from build123d import *

# Parameters (mm, degrees)
SKETCH1_R           = 2
SKETCH1_R_2         = 1.95
SKETCH1_R_3         = 1.5
BOSS_EXTRUDE1_DEPTH = 5
SKETCH2_R           = 1.5
SKETCH2_R_2         = 1.95
SKETCH2_R_3         = 2
SKETCH2_W           = 36
SKETCH2_H           = 70
CUT_EXTRUDE1_DEPTH  = 142.509716981
FILLET1_R           = 2


with BuildPart() as part:
    # Sketch1 → Boss-Extrude1 (new body)
    with BuildSketch(Plane.XY):
        with BuildLine():
            Line((-90, 100), (-70, 100))
            Line((-70, 100), (-14.884168151, 68.505238943))
            ThreePointArc((-14.884168151, 68.505238943), (0, 64.552533207), (14.884168151, 68.505238943))
            Line((14.884168151, 68.505238943), (70, 100))
            Line((70, 100), (90, 100))
            ThreePointArc((90, 100), (97.071067812, 97.071067812), (100, 90))
            Line((100, 90), (100, 29))
            Line((100, 29), (93.372317414, 9.7797205))
            ThreePointArc((93.372317414, 9.7797205), (91.733506862, 0), (93.372317414, -9.7797205))
            Line((93.372317414, -9.7797205), (100, -29))
            Line((100, -29), (100, -90))
            ThreePointArc((100, -90), (97.071067812, -97.071067812), (90, -100))
            Line((90, -100), (70, -100))
            Line((70, -100), (14.884168151, -68.505238943))
            ThreePointArc((14.884168151, -68.505238943), (0, -64.552533207), (-14.884168151, -68.505238943))
            Line((-14.884168151, -68.505238943), (-70, -100))
            Line((-70, -100), (-90, -100))
            ThreePointArc((-90, -100), (-97.071067812, -97.071067812), (-100, -90))
            Line((-100, -90), (-100, -29))
            Line((-100, -29), (-93.372317414, -9.7797205))
            ThreePointArc((-93.372317414, -9.7797205), (-91.733506862, 0), (-93.372317414, 9.7797205))
            Line((-93.372317414, 9.7797205), (-100, 29))
            Line((-100, 29), (-100, 90))
            ThreePointArc((-100, 90), (-97.071067812, 97.071067812), (-90, 100))
        make_face()
        with Locations((-91.923881554, 91.923881554)):
            Circle(SKETCH1_R, mode=Mode.SUBTRACT)
        with Locations((91.923881554, 91.923881554)):
            Circle(SKETCH1_R, mode=Mode.SUBTRACT)
        with Locations((91.923881554, -91.923881554)):
            Circle(SKETCH1_R, mode=Mode.SUBTRACT)
        with Locations((-91.923881554, -91.923881554)):
            Circle(SKETCH1_R, mode=Mode.SUBTRACT)
        with Locations((58, 29)):
            Circle(SKETCH1_R_2, mode=Mode.SUBTRACT)
        with Locations((82, 29)):
            Circle(SKETCH1_R_2, mode=Mode.SUBTRACT)
        with Locations((58, 11)):
            Circle(SKETCH1_R_2, mode=Mode.SUBTRACT)
        with Locations((82, 11)):
            Circle(SKETCH1_R_2, mode=Mode.SUBTRACT)
        with Locations((58, -11)):
            Circle(SKETCH1_R_2, mode=Mode.SUBTRACT)
        with Locations((58, -29)):
            Circle(SKETCH1_R_2, mode=Mode.SUBTRACT)
        with Locations((82, -11)):
            Circle(SKETCH1_R_2, mode=Mode.SUBTRACT)
        with Locations((82, -29)):
            Circle(SKETCH1_R_2, mode=Mode.SUBTRACT)
        with Locations((-82, 29)):
            Circle(SKETCH1_R_2, mode=Mode.SUBTRACT)
        with Locations((-58, 29)):
            Circle(SKETCH1_R_2, mode=Mode.SUBTRACT)
        with Locations((-82, 11)):
            Circle(SKETCH1_R_2, mode=Mode.SUBTRACT)
        with Locations((-58, 11)):
            Circle(SKETCH1_R_2, mode=Mode.SUBTRACT)
        with Locations((-82, -11)):
            Circle(SKETCH1_R_2, mode=Mode.SUBTRACT)
        with Locations((-82, -29)):
            Circle(SKETCH1_R_2, mode=Mode.SUBTRACT)
        with Locations((-58, -11)):
            Circle(SKETCH1_R_2, mode=Mode.SUBTRACT)
        with Locations((-58, -29)):
            Circle(SKETCH1_R_2, mode=Mode.SUBTRACT)
        with Locations((-6, 10)):
            Circle(SKETCH1_R_3, mode=Mode.SUBTRACT)
        with Locations((6, 10)):
            Circle(SKETCH1_R_3, mode=Mode.SUBTRACT)
        with Locations((-6, -10)):
            Circle(SKETCH1_R_3, mode=Mode.SUBTRACT)
        with Locations((6, -10)):
            Circle(SKETCH1_R_3, mode=Mode.SUBTRACT)
    extrude(amount=BOSS_EXTRUDE1_DEPTH)

    # Sketch2 → Cut-Extrude1 (cut, through all)
    with BuildSketch(Plane.XY.offset(5)):
        with BuildLine():
            Line((100, 29), (100, 90))
            ThreePointArc((100, 90), (97.071067812, 97.071067812), (90, 100))
            Line((90, 100), (70, 100))
            Line((70, 100), (14.884168151, 68.505238943))
            ThreePointArc((14.884168151, 68.505238943), (0, 64.552533207), (-14.884168151, 68.505238943))
            Line((-14.884168151, 68.505238943), (-70, 100))
            Line((-70, 100), (-90, 100))
            ThreePointArc((-90, 100), (-97.071067812, 97.071067812), (-100, 90))
            Line((-100, 90), (-100, 29))
            Line((-100, 29), (-93.372317414, 9.7797205))
            ThreePointArc((-93.372317414, 9.7797205), (-91.733506862, 0), (-93.372317414, -9.7797205))
            Line((-93.372317414, -9.7797205), (-100, -29))
            Line((-100, -29), (-100, -90))
            ThreePointArc((-100, -90), (-97.071067812, -97.071067812), (-90, -100))
            Line((-90, -100), (-70, -100))
            Line((-70, -100), (-14.884168151, -68.505238943))
            ThreePointArc((-14.884168151, -68.505238943), (0, -64.552533207), (14.884168151, -68.505238943))
            Line((14.884168151, -68.505238943), (70, -100))
            Line((70, -100), (90, -100))
            ThreePointArc((90, -100), (97.071067812, -97.071067812), (100, -90))
            Line((100, -90), (100, -29))
            Line((100, -29), (93.372317414, -9.7797205))
            ThreePointArc((93.372317414, -9.7797205), (91.733506862, 0), (93.372317414, 9.7797205))
            Line((93.372317414, 9.7797205), (100, 29))
        make_face()
        with Locations((-6, 10)):
            Circle(SKETCH2_R, mode=Mode.SUBTRACT)
        with Locations((58, -11)):
            Circle(SKETCH2_R_2, mode=Mode.SUBTRACT)
        with Locations((58, 29)):
            Circle(SKETCH2_R_2, mode=Mode.SUBTRACT)
        with Locations((-91.923881554, 91.923881554)):
            Circle(SKETCH2_R_3, mode=Mode.SUBTRACT)
        with Locations((91.923881554, 91.923881554)):
            Circle(SKETCH2_R_3, mode=Mode.SUBTRACT)
        with Locations((82, 29)):
            Circle(SKETCH2_R_2, mode=Mode.SUBTRACT)
        with Locations((58, -29)):
            Circle(SKETCH2_R_2, mode=Mode.SUBTRACT)
        with Locations((6, 10)):
            Circle(SKETCH2_R, mode=Mode.SUBTRACT)
        with Locations((6, -10)):
            Circle(SKETCH2_R, mode=Mode.SUBTRACT)
        with Locations((82, -29)):
            Circle(SKETCH2_R_2, mode=Mode.SUBTRACT)
        with Locations((82, 11)):
            Circle(SKETCH2_R_2, mode=Mode.SUBTRACT)
        with Locations((-70, 0)):
            Rectangle(SKETCH2_W, SKETCH2_H, mode=Mode.SUBTRACT)
    extrude(amount=-CUT_EXTRUDE1_DEPTH, mode=Mode.SUBTRACT)

    # Fillet1
    fillet1_edges = [part.edges().sort_by_distance(p)[0] for p in [
        (-52, -35, 2.5),
        (-52, 35, 2.5),
        (-88, 35, 2.5),
        (-88, -35, 2.5),
    ]]
    fillet(fillet1_edges, radius=FILLET1_R)


solid = part.part
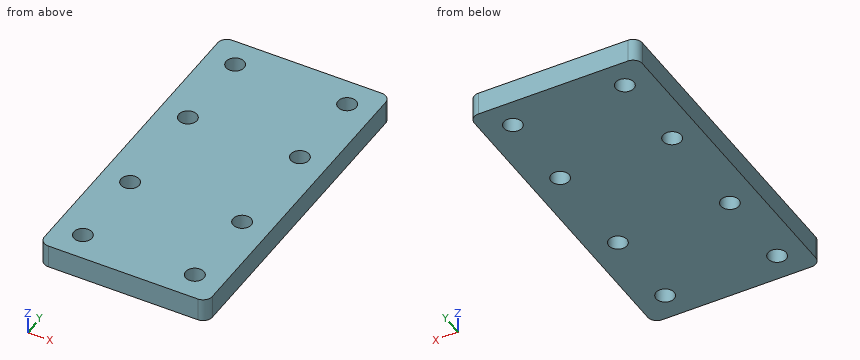
For this review, take the finished solid that the model builds, in its own axes (mm). Give positions to 0.01 mm unless a question says otherwise; leave off trailing zeros. Loops run counter-clockwise (first coordinate to the right, second up) from the corner with the lowest first, then second, coordinate; pieces in that order, holes last. Notation, with made-up numbers: (54, -9) - (107, -9) arc R17 ccw to (107, 5) - close; hole circle Ø10 at (48.25, 87). An arc over 180 degrees is marked (long way). Write each question's results on one line, items separated by ' | '.
(1) Take a section at A-A (x = -82). Give the boundary of the cut face in (y, z), then the cut area to 3 significant figures.
Conclusion:
outline: (-35, 0) - (-30.95, 0) - (-30.95, 5) - (-35, 5) - close; (-27.05, 0) - (-12.95, 0) - (-12.95, 5) - (-27.05, 5) - close; (-9.05, 0) - (9.05, 0) - (9.05, 5) - (-9.05, 5) - close; (12.95, 0) - (27.05, 0) - (27.05, 5) - (12.95, 5) - close; (30.95, 0) - (35, 0) - (35, 5) - (30.95, 5) - close | area: 272 mm^2
(2) For line 1 along Y through (x, z) = (-58, 3.2); line 2 along Y through (x, z) = (-81, 0.4), list the stretches that pass through material, from the lowest coordinate up.
Conclusion:
line 1: -35 to -30.95, -27.05 to -12.95, -9.05 to 9.05, 12.95 to 27.05, 30.95 to 35 | line 2: -35 to -30.67, -27.33 to -12.67, -9.33 to 9.33, 12.67 to 27.33, 30.67 to 35
(3) For pin 1 Ø6 at (x, y) = (-82, 11) entering from -Z, flat-tipped, find the tip position at first contact; note if it passes through.
Conclusion:
pin 1: z = 0
(4) Take a section at C-C (z = 4.2). State how many separate pieces and enclosed holes the cut face has, then the cut area to 3 significant figures.
Conclusion:
separate pieces: 1 | enclosed holes: 8 | area: 2,420 mm^2
(5) Take a section at B-B (y = 11). Give the boundary of the cut face in (x, z).
Conclusion:
outline: (-88, 0) - (-83.95, 0) - (-83.95, 5) - (-88, 5) - close; (-80.05, 0) - (-59.95, 0) - (-59.95, 5) - (-80.05, 5) - close; (-56.05, 0) - (-52, 0) - (-52, 5) - (-56.05, 5) - close
